Autodesk Fusion 360 part; units mm, degrees
sketch "Sketch1" plane through (0, 0, 0) normal (0, 0, 1) x (1, 0, 0)
  line L0 (0, 0) -> (75, 0)
  line L1 (75, 0) -> (75, 81)
  line L2 (75, 81) -> (0, 81)
  line L3 (0, 81) -> (0, 0)
  dimension "d1" = 81
  dimension "d2" = 75
extrude "Extrude1" add sketch "Sketch1" along normal blind 4
sketch "Sketch2" plane through (0, 0, 0) normal (0, 0, -1) x (1, 0, 0)
  line L0 (0, 0) -> (0, -81)
  line L1 (0, -81) -> (75, -81)
  line L2 (75, -81) -> (75, 0)
  line L3 (75, 0) -> (0, 0)
  line L4 (72.95, -78.95) -> (2.05, -78.95)
  line L5 (2.05, -78.95) -> (2.05, -2.05)
  line L6 (2.05, -2.05) -> (72.95, -2.05)
  line L7 (72.95, -2.05) -> (72.95, -78.95)
  dimension "d6" = 2.05
  dimension "d7" = 2.05
  dimension "d8" = 2.05
  dimension "d9" = 2.05
extrude "Extrude2" add sketch "Sketch2" along normal blind 2 contours L4 L5 L6 L7
sketch "Sketch3" plane through (0, 0, 4) normal (0, 0, 1) x (-1, 0, 0)
  line L0 (0, -81) -> (0, 0)
  line L1 (0, 0) -> (-75, 0)
  line L2 (-75, 0) -> (-75, -81)
  line L3 (-75, -81) -> (0, -81)
  circle A0 centre (-6, -6) radius 2.875
  circle A1 centre (-69, -6) radius 2.875
  circle A2 centre (-25, -75) radius 2.875
  dimension "d12" = 25
  dimension "d13" = 5.75
  dimension "d14" = 6
  dimension "d15" = 6
  dimension "d16" = 6
  dimension "d17" = 6
  dimension "d18" = 6
  dimension "d19" = 5.75
  dimension "d20" = 5.75
extrude "Extrude3" cut sketch "Sketch3" against normal blind 3 contours A0 | A1 | A2
sketch "Sketch4" plane through (0, 0, 4) normal (0, 0, 1) x (-1, 0, 0)
  circle A0 centre (-25, -75) radius 2.875
  circle A1 centre (-6, -6) radius 2.875
  circle A2 centre (-69, -6) radius 2.875
  line L0 (0, -81) -> (0, 0)
  line L1 (0, 0) -> (-75, 0)
  line L2 (-75, 0) -> (-75, -81)
  line L3 (-75, -81) -> (0, -81)
  circle A3 centre (-6, -6) radius 1.55
  circle A4 centre (-69, -6) radius 1.55
  circle A5 centre (-25, -75) radius 1.55
  dimension "d23" = 3.1
  dimension "d24" = 3.1
  dimension "d25" = 3.1
extrude "Extrude4" cut sketch "Sketch4" against normal blind 16 contours A3 | A4 | A5
sketch "Sketch5" plane through (0, 0, 4) normal (0, 0, 1) x (-1, 0, 0)
  circle A0 centre (-25, -75) radius 2.875
  circle A1 centre (-6, -6) radius 2.875
  circle A2 centre (-69, -6) radius 2.875
  line L0 (0, -81) -> (0, 0)
  line L1 (0, 0) -> (-75, 0)
  line L2 (-75, 0) -> (-75, -81)
  line L3 (-75, -81) -> (0, -81)
  line L4 (-69, -66) -> (-6, -66)
  line L5 (-6, -66) -> (-6, -43)
  line L6 (-6, -43) -> (-69, -43)
  line L7 (-69, -43) -> (-69, -66)
  line L8 (-69, -38) -> (-6, -38)
  line L9 (-6, -38) -> (-6, -15)
  line L10 (-6, -15) -> (-69, -15)
  line L11 (-69, -15) -> (-69, -38)
  dimension "d28" = 23
  dimension "d29" = 15
  dimension "d30" = 23
  dimension "d31" = 15
  dimension "d32" = 6
  dimension "d33" = 6
  dimension "d34" = 6
  dimension "d35" = 6
extrude "Extrude5" cut sketch "Sketch5" against normal blind 2 contours L4 L5 L6 L7 | L8 L9 L10 L11
The model under review builds one solid part; all positions refer to its coordinate system, in mm. A direction names the side the tool comes from. Round coordinates to 2 decimals unless told otherwise and drop trailing zeros. Loops run counter-clockwise (first coordinate to the right, second up) from the corner with the lowest first, then second, coordinate; pieces in that order, holes last. Notation, with made-up numbers: M 64.5,-25.75 L 68.5,-25.75 A18 cw 68.5,-19.75 Z; hole C 27.25,42.5 d9. An arc over 180 degrees is marked long. Put each result on its own line as item: value.
Q1. Consider section A-A, the plane y = 6. Give the boundary of the cut face in (x, z) (3 decimals).
Result set:
outline: M 0,0 L 2.05,0 L 2.05,-2 L 4.45,-2 L 4.45,1 L 3.125,1 L 3.125,4 L 0,4 Z; M 7.55,-2 L 67.45,-2 L 67.45,1 L 66.125,1 L 66.125,4 L 8.875,4 L 8.875,1 L 7.55,1 Z; M 70.55,-2 L 72.95,-2 L 72.95,0 L 75,0 L 75,4 L 71.875,4 L 71.875,1 L 70.55,1 Z
Q2. Consider section D-D, the plane x = 54. Give the boundary of the cut face in (y, z).
Result set:
outline: M 0,0 L 2.05,0 L 2.05,-2 L 78.95,-2 L 78.95,0 L 81,0 L 81,4 L 66,4 L 66,2 L 43,2 L 43,4 L 38,4 L 38,2 L 15,2 L 15,4 L 0,4 Z
Q3. Consider section B-B, the plane y = 75. Give the boundary of the cut face in (x, z) (3 decimals), then the cut area to 3 significant figures.
Result set:
outline: M 0,0 L 2.05,0 L 2.05,-2 L 23.45,-2 L 23.45,1 L 22.125,1 L 22.125,4 L 0,4 Z; M 26.55,-2 L 72.95,-2 L 72.95,0 L 75,0 L 75,4 L 27.875,4 L 27.875,1 L 26.55,1 Z
area: 415 mm²
Q4. For pin 1 (11.5 mm diameter, centred on x = 47.5, y = 27, fed in from +Z); pin 2 (1.7 mm diameter, centred on x = 7, y = 5, fed in from +Z); pin 3 (3.5 mm diameter, centred on x = 25, y = 75, fed in from -Z); pin 4 (1 mm diameter, centred on x = 40, z = -1.5, fed in from +Y), all flat-tipped, find the tip position at first contact; note any pin that passes through.
Result set:
pin 1: stops at z = 2
pin 2: stops at z = 1
pin 3: stops at z = -2
pin 4: stops at y = 78.95
Q5. Mouldability with a two-part tool opening along Z and no side actions: class faces 1 (the flat face through (37, 40, -2)), 2 (the flat face through (69, 26, 3)), 3 (the flat face through (23.76, 76.24, 1)) as released by +Z, released by -Z, zero draft, split by the parting line, or undercut.
Result set:
face 1: released by -Z
face 2: zero draft
face 3: released by +Z
Q6. Machinability: for faces 4 (the flat face through (6, 55, 3)), 5 (the flat face through (2.05, 41, -1)), 6 (the flat face through (37, 2.05, -1)), which of the approach directions +Z, -Z, +X, -X, +Y, -Y give a long, thin tool a straight path to every point of the face, cutting with its end or side? Answer none if there is none.
Result set:
face 4: +Z
face 5: -Z, -X, +Y, -Y
face 6: -Z, +X, -X, -Y
Q7. To check wall thickness, follow L1, parallel to Y at x = 37, z = 3.4; L2, parallel to X at y = 6, z = 1.95 (3 decimals); L3, parallel to Y at x = 25, z = 2.9 (3 decimals). State the ranges of each line that lie inside material, in increasing order.
Result set:
L1: y = 0 to 15, 38 to 43, 66 to 81
L2: x = 0 to 3.125, 8.875 to 66.125, 71.875 to 75
L3: y = 0 to 15, 38 to 43, 66 to 72.125, 77.875 to 81
Q8. Consider section C-C, the plane z = 3. Give the boundary of the cut face in (x, y) (3 decimals), then the cut area to 3 significant figures.
Result set:
outline: M 0,0 L 75,0 L 75,81 L 0,81 Z; hole C 6,6 d5.75; hole M 6,15 L 69,15 L 69,38 L 6,38 Z; hole M 6,43 L 69,43 L 69,66 L 6,66 Z; hole C 25,75 d5.75; hole C 69,6 d5.75
area: 3,100 mm²
